```python
from build123d import *

# Parameters (mm, degrees)
F0_W     = 152.4
F0_H     = 457.2
F1_DEPTH = 50.8
F2_W     = 152.4
F2_H     = 54.4068123519
F3_DEPTH = 152.4
F4_R     = 76.19999
F5_R     = 45.72
F5_R_2   = 53.4879372825
F6_DEPTH = 50.801
F7_R     = 25.4
F8_DEPTH = 54.4078123519
F9_SIZE  = 38.1


# Not quite as in the source:
# - a fillet or chamfer is up to 0.001 mm smaller than in the source, because OpenCascade refuses the exact size


with BuildPart() as f1:
    # F0 (on Top) → F1 (new body)
    with BuildSketch(Plane.XY):
        with Locations((39.8436626315, 216.4812246025)):
            Rectangle(F0_W, F0_H)
    extrude(amount=F1_DEPTH)

    # F2 (on face) → F3 (join)
    with BuildSketch(Plane(origin=(0, 0, 0), x_dir=(1, 0, 0), z_dir=(0, 0, -1))):
        with Locations((39.8436626315, -417.8778184265)):
            Rectangle(F2_W, F2_H)
    extrude(amount=F3_DEPTH)

    # F4 (radius 76.2 in the source; OpenCascade refuses exactly that, so slightly less here)
    f4_edges = [f1.edges().sort_by_distance(p)[0] for p in [
        (116.043663, 417.877818, -152.4),
        (-36.356337, 417.877818, -152.4),
    ]]
    fillet(f4_edges, radius=F4_R)

    # F5 (on face) → F6 (cut, through all)
    with BuildSketch(Plane(origin=(0, 0, 0), x_dir=(1, 0, 0), z_dir=(0, 0, -1))):
        with Locations((39.8436626315, -279.9812246025)):
            Circle(F5_R)
        with Locations((39.8436626315, -114.8812246025)):
            Circle(F5_R_2)
    extrude(amount=-F6_DEPTH, mode=Mode.SUBTRACT)

    # F7 (on face) → F8 (cut, through all)
    with BuildSketch(Plane.XZ.offset(-390.6744122505)):
        with Locations((39.8436626315, -76.2)):
            Circle(F7_R)
    extrude(amount=-F8_DEPTH, mode=Mode.SUBTRACT)

    # F9
    f9_edges = [f1.edges().sort_by_distance(p)[0] for p in [
        (116.043663, -12.118775, 25.4),
        (-36.356337, -12.118775, 25.4),
    ]]
    chamfer(f9_edges, length=F9_SIZE)


solid = f1.part
```
Part model, mm, in its own coordinate system. A direction names the side the tool comes from. Give positions to 0.01 mm unless a question says otherwise; leave off trailing zeros. Write each loop counter-clockwise with the first axis right and the second up, starting at its lowest first coordinate (ties: lowest second). Pieces come first, ordered by that corner, then holes. Notation, with made-up numbers: (-5, 10.25) -> (22, 10.25) arc R20 ccw to (22, 21.25) -> close; hole circle Ø2 at (6, 53.5). An arc over 180 degrees is marked (long way). Put each result on its own line as item: value. Start each with the question number.
Item 1: Cut at B-B (z = -90.5). List the corners of the cut face in (x, y), then the cut area to 3 significant figures.
Item 2: Cut at D-D (z = -26.5). List the corners of the cut face in (x, y), then the cut area to 3 significant figures.
Item 3: Which spindle directions (+Z, -Z, +X, -X, +Y, -Y) get a long thin tool onto all of the face, cutting with end or side? Do faces 4 (the face through (39, 390.674, -41)), 5 (the face through (39, 220, 50.8)). Say none if no direction does.
Item 4: Cut at C-C (y = 287.5). List the corners of the cut face in (x, z), then the cut area to 3 significant figures.
Item 5: Pull direction X, two halves, no side cores. Call faces 1 (the face through (116.044, 238, 16)), 2 (the face through (34.337, 417.497, -100.996)), 3 (the face through (39, -12.119, 25)): pulls with the +X half, pulls with the -X half, needs draft (parallel to the pull), parting line crosses it, or undercut.
Item 6: Wall check: L1, parallel to X at y = 429, z = -76; L2, parallel to Y at x = 62, z = 34.5; L3, parallel to Y at x = 12, z = -19. Give the ranges that are in metal, low to high. Write a range as [from, to].
Item 7: Pin check, flat tips, straight feed: pin 1 Ø1.5 at (x, z) = (70, -77) entering from -Y; pin 2 Ø5 at (x, y) = (58, 235) entering from -Z. Stop position of each tip, or through.
Answer list:
1. outline: (-35, 390.67) -> (18.85, 390.67) -> (18.85, 445.08) -> (-35, 445.08) -> close; (60.84, 390.67) -> (114.69, 390.67) -> (114.69, 445.08) -> (60.84, 445.08) -> close
1. area: 5,860 mm2
2. outline: (-36.36, 390.67) -> (116.04, 390.67) -> (116.04, 445.08) -> (-36.36, 445.08) -> close
2. area: 8,290 mm2
3. face 4: -Z, +X, -X, -Y
3. face 5: +Z, +X, -X, +Y, -Y
4. outline: (-36.36, 0) -> (-5.25, 0) -> (-5.25, 50.8) -> (-36.36, 50.8) -> close; (84.94, 0) -> (116.04, 0) -> (116.04, 50.8) -> (84.94, 50.8) -> close
4. area: 3,160 mm2
5. face 1: pulls with the +X half
5. face 2: undercut
5. face 3: needs draft
6. L1: x = [-36.36, 14.44], [65.24, 116.04]
6. L2: y = [-12.12, 66.2], [163.56, 239.99], [319.97, 445.08]
6. L3: y = [390.67, 445.08]
7. pin 1: stops at y = 390.67
7. pin 2: stops at z = 0
